The model under review builds one solid part; all positions refer to its coordinate system, in mm. Face numbers are marked on the shaded views. Round coordinates to 2 decimals unless told otherwise and drop trailing zeros. Loops run counter-clockwise (first coordinate to the right, second up) from the corner with the lowest first, then second, coordinate; pieces in that order, holes last. Notation, with made-up numbers: (26, 65) -> (72, 65) arc R13 ccw to (72, 71) -> close; hole circle Ø5 at (12, 56). An arc over 180 degrees is marked (long way). Use a Markdown table: item, result. Add a question column.
1) Consider section C-C on y = -25.4. Give the boundary of the cut face in (x, z).
2) Mouldability with a two-part tool opening along Y and no side actions: class the marked faces 1, 2, 3 and 4 as released by +Y, released by -Y, zero draft, split by the parting line, or undercut.
3) Consider section B-B on x = 25.4. Give the boundary of the cut face in (y, z).
4) Consider section A-A on z = 31.5. Give the boundary of the cut face in (x, y), plus the area to 3 significant figures.
5) Consider section D-D on z = 3.5. Give the boundary of the cut face in (x, y).
6) Wall thickness on probe 1 along Y at (x, z) = (46.5, 27.5); probe 2 along X at (y, z) = (-25.4, 3.25); probe 3 along Y at (x, z) = (25, 4): over which ranges is each line inside the solid? List them lowest first.
7) Insertion check: pin 1 (15 mm diameter, centred on x = 25.4, y = -25.4, fed in from +Z). The pin has a flat end and moves straight along its axis. Give the tip position at first contact, or say it passes through.
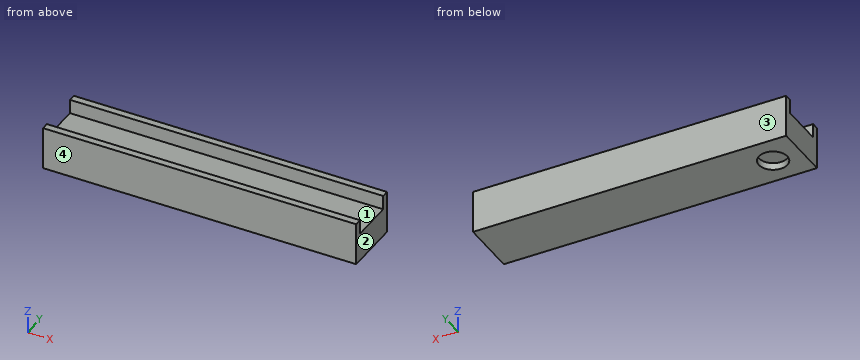
from build123d import *

# Parameters (mm, degrees)
F0_W     = 685.8
F0_H     = 25.4
F1_DEPTH = 50.8
F2_W     = 685.8
F2_H     = 6.35
F3_DEPTH = 12.7
F4_R     = 12.7
F5_DEPTH = 6.35
F6_R     = 12.7
F7_DEPTH = 6.35
F8_W     = 406.4
F8_H     = 38.1
F9_DEPTH = 50.8


with BuildPart() as f1:
    # F0 (on Front) → F1 (new body)
    with BuildSketch(Plane.XZ):
        with Locations((342.9, 12.7)):
            Rectangle(F0_W, F0_H)
    extrude(amount=F1_DEPTH)

    # F2 (on face) → F3 (join)
    with BuildSketch(Plane.XY.offset(25.4)):
        with Locations((342.9, -47.625)):
            Rectangle(F2_W, F2_H)
        with Locations((342.9, -3.175)):
            Rectangle(F2_W, F2_H)
    extrude(amount=F3_DEPTH)

    # F4 (on face) → F5 (cut)
    with BuildSketch(Plane(origin=(0, 0, 0), x_dir=(1, 0, 0), z_dir=(0, 0, -1))):
        with Locations((342.9, 25.4)):
            Circle(F4_R)
    extrude(amount=-F5_DEPTH, mode=Mode.SUBTRACT)

    # F6 (on face) → F7 (cut)
    with BuildSketch(Plane(origin=(0, 0, 0), x_dir=(1, 0, 0), z_dir=(0, 0, -1))):
        with Locations((25.4, 25.4)):
            Circle(F6_R)
        with Locations((660.4, 25.4)):
            Circle(F6_R)
    extrude(amount=-F7_DEPTH, mode=Mode.SUBTRACT)

    # F8 (on face) → F9 (cut)
    with BuildSketch(Plane.XZ.offset(50.8)):
        with Locations((482.6, 19.05)):
            Rectangle(F8_W, F8_H)
    extrude(amount=-F9_DEPTH, mode=Mode.SUBTRACT)


solid = f1.part
Result set:
| question | item | result |
|---|---|---|
| 1 | outline | (0, 0) -> (12.7, 0) -> (12.7, 6.35) -> (38.1, 6.35) -> (38.1, 0) -> (279.4, 0) -> (279.4, 25.4) -> (0, 25.4) -> close |
| 2 | face 1 | undercut |
| 2 | face 2 | zero draft |
| 2 | face 3 | released by +Y |
| 2 | face 4 | released by -Y |
| 3 | outline | (-50.8, 0) -> (-38.1, 0) -> (-38.1, 6.35) -> (-12.7, 6.35) -> (-12.7, 0) -> (0, 0) -> (0, 38.1) -> (-6.35, 38.1) -> (-6.35, 25.4) -> (-44.45, 25.4) -> (-44.45, 38.1) -> (-50.8, 38.1) -> close |
| 4 | outline | (0, -50.8) -> (279.4, -50.8) -> (279.4, -44.45) -> (0, -44.45) -> close; (0, -6.35) -> (279.4, -6.35) -> (279.4, 0) -> (0, 0) -> close |
| 4 | area | 3,550 mm2 |
| 5 | outline | (0, -50.8) -> (279.4, -50.8) -> (279.4, 0) -> (0, 0) -> close; hole circle Ø25.4 at (25.4, -25.4) |
| 6 | probe 1 | -50.8 to -44.45, -6.35 to 0 |
| 6 | probe 2 | 0 to 12.7, 38.1 to 279.4 |
| 6 | probe 3 | -50.8 to -38.09, -12.71 to 0 |
| 7 | pin 1 | z = 25.4 |
